Part model, mm, in its own coordinate system. A direction names the side the tool comes from. Round coordinates to 2 decimals unless told otherwise and drop trailing zeros. Write each loop counter-clockwise with the first axis right and the second up, starting at its lowest first coordinate (ties: lowest second). Pieces come first, ordered by that corner, then holes. Notation, with made-up numbers: M -4,39.25 L 42,39.25 A22 cw 42,78.25 Z; hole C -22.75,9 d10. An arc over 180 degrees is marked long. Use a Markdown table: item, result. Add a question column.
1) Slice it at C-C on z = -55.5. Write the cut outline in (x, y), plus the area to 3 significant figures.
2) Wall check: probe 1 along X at (y, z) = (97.5, -117); probe 2 along Y at (x, z) = (-33.5, -18.5); probe 3 along Y at (x, z) = (-47, 9). Give the ranges that are in metal, low to high.
3) Slice it at B-B on x = 37.5. Write the cut outline in (y, z).
4) Two-plate mould, pull along X, no slides. Class faces 1 (the face through (-37.134, 50, -46)), 2 (the face through (10.727, 29.723, -187)), 3 (the face through (-55.291, 51.511, -141.795)), 4 (the face through (7, 50, -124.033)): released by +X, released by -X, zero draft, split by the parting line, or undercut.
5) Which spindle directions (+Z, -Z, +X, -X, +Y, -Y) get a long thin tool onto all of the face, cutting with end or side? Do faces 5 (the face through (5.44, 31.65, -27.32)), 6 (the face through (-62.534, 50, -44)). Say none if no direction does.
6) Slice it at D-D on y = 14. Write the cut outline in (x, z).
7) Drop flat-ended pins along their axis: P1, Ø4, axis at x = 49, y = 52.5, coming from the -Z side; P2, Ø6, axis at x = 43, y = 61.5, coming from the +Z side; P3, Ø1, axis at y = 33, z = -171.5, coming from the -X side. Give the stop position or say it passes through.
8) Slice it at A-A on y = 50.8. Write the cut outline in (x, z), plus the area to 3 significant figures.
```python
from build123d import *

# Parameters (mm, degrees)
BOSS_EXTRUDE1_DEPTH = 101.6
BOSS_EXTRUDE2_REACH = 113.76
SKETCH3_R           = 21.59
SKETCH4_R           = 21.59
BOSS_EXTRUDE3_DEPTH = 76.2
FILLET1_R           = 25.4
FILLET2_R           = 25.4
FILLET4_R           = 25.4
FILLET5_R           = 25.4


with BuildPart() as part:
    # Sketch1 → Boss-Extrude1 (new body)
    with BuildSketch(Plane(origin=(0, 0, 0), x_dir=(1, 0, 0), z_dir=(0, 1, 0))):
        Polygon((-37.133661193, -33.44672), (-62.533661193, -33.44672), (-62.533661193, 149.43328), (74.626338807, 149.43328), (74.626338807, -33.44672), (49.226338807, -33.44672), (49.226338807, 124.03328), (-37.133661193, 124.03328), align=None)
    extrude(amount=BOSS_EXTRUDE1_DEPTH)

    # Sketch3 → Boss-Extrude2 (add, up to next)
    with BuildSketch(Plane(origin=(-37.133661193, 0, 0), x_dir=(0, 0, -1), z_dir=(1, 0, 0)), mode=Mode.PRIVATE) as boss_extrude2_sk1:
        with Locations((17.35328, 50.8)):
            Circle(SKETCH3_R)
    boss_extrude2_tool1 = extrude(boss_extrude2_sk1.sketch, amount=BOSS_EXTRUDE2_REACH, mode=Mode.PRIVATE) - part.part
    add(boss_extrude2_tool1.solids().sort_by_distance((-37.133661, 50.8, -17.35328))[0])

    # Sketch4 → Boss-Extrude3 (add)
    with BuildSketch(Plane(origin=(0, 0, -149.43328), x_dir=(-1, 0, 0), z_dir=(0, 0, -1))):
        with Locations((-6.046338807, 50.8)):
            Circle(SKETCH4_R)
    extrude(amount=BOSS_EXTRUDE3_DEPTH)

    # Fillet1
    fillet1_edges = [part.edges().sort_by_distance(p)[0] for p in [
        (-49.833661193, 101.6, 33.44672),
        (-49.833661193, 0, 33.44672),
    ]]
    fillet(fillet1_edges, radius=FILLET1_R)

    # Fillet2
    fillet2_edges = [part.edges().sort_by_distance(p)[0] for p in [
        (-62.533661193, 50.8, -149.43328),
    ]]
    fillet(fillet2_edges, radius=FILLET2_R)

    # Fillet4
    fillet4_edges = [part.edges().sort_by_distance(p)[0] for p in [
        (61.926338807, 0, 33.44672),
        (61.926338807, 101.6, 33.44672),
    ]]
    fillet(fillet4_edges, radius=FILLET4_R)

    # Fillet5
    fillet5_edges = [part.edges().sort_by_distance(p)[0] for p in [
        (74.626338807, 50.8, -149.43328),
    ]]
    fillet(fillet5_edges, radius=FILLET5_R)


solid = part.part
```
Entries:
| question | item | result |
|---|---|---|
| 1 | outline | M -62.53,0 L -37.13,0 L -37.13,101.6 L -62.53,101.6 Z; M 49.23,0 L 74.63,0 L 74.63,101.6 L 49.23,101.6 Z |
| 1 | area | 5,160 mm^2 |
| 2 | probe 1 | x = -62.53 to -37.13, 49.23 to 74.63 |
| 2 | probe 2 | y = 29.24 to 72.36 |
| 2 | probe 3 | y = 0.02 to 101.58 |
| 3 | outline | M 0,-149.43 L 101.6,-149.43 L 101.6,-124.03 L 0,-124.03 Z; C 50.8,-17.35 d43.18 |
| 4 | face 1 | undercut |
| 4 | face 2 | split by the parting line |
| 4 | face 3 | released by -X |
| 4 | face 4 | undercut |
| 5 | face 5 | none |
| 5 | face 6 | +Z, -Z, -X, +Y, -Y |
| 6 | outline | M -62.53,-124.03 A25.4 ccw -37.13,-149.43 L 49.23,-149.43 A25.4 ccw 74.63,-124.03 L 74.63,30.74 L 49.23,30.74 L 49.23,-124.03 L -37.13,-124.03 L -37.13,30.74 L -62.53,30.74 Z |
| 7 | P1 | stops at z = -149.43 |
| 7 | P2 | stops at z = 2.82 |
| 7 | P3 | stops at x = -6.87 |
| 8 | outline | M -62.53,-124.03 A25.4 ccw -37.13,-149.43 L -15.54,-149.43 L -15.54,-225.63 L 27.64,-225.63 L 27.64,-149.43 L 49.23,-149.43 A25.4 ccw 74.63,-124.03 L 74.63,33.45 L 49.23,33.45 L 49.23,4.24 L -37.13,4.24 L -37.13,33.45 L -62.53,33.45 Z; hole M -37.13,-124.03 L 49.23,-124.03 L 49.23,-38.94 L -37.13,-38.94 Z |
| 8 | area | 18,200 mm^2 |
